Geometry check sheet. Reference: the model listing, model coordinates, mm. Face numbers are marked on the shaded views. A direction names the side the tool comes from. Give positions to 0.01 mm unless a question says otherwise; leave off trailing zeros. Loops run counter-clockwise (first coordinate to the right, second up) from the corner with the lowest first, then second, coordinate; pieces in that order, holes last. Notation, with made-up numbers: (74, 11.5) -> (133, 11.5) arc R22 cw to (133, 20.5) -> close; hole circle Ø3 at (80, 74). An arc over 180 degrees is marked (long way). One line per item, written item: value. Start each with the question number.
(1) Tool access check on the marked faces 1, 2 and 3. Record the directions out of +Z, -Z, +X, -X, +Y, -Y that give a thin tool (end or side, any length) a straight path to the whole face; none if there is none.
(2) Scan lines: line 1 along Z through (x, y) = (25.41, 0.5); line 2 along X through (y, z) = (1.1, 41.59); line 3 along Y through (x, z) = (-19, 34.5). Record each from-to range of solid material in increasing order. Write a range as from..to.
(3) Sectioned sample at C-C, the plane z = -8.5. Record the cut outline in (x, y), then the cut area to 3 significant figures.
(4) Sectioned sample at D-D, the plane x = -7. Record the cut outline in (y, z), then the cut area to 3 significant figures.
(5) Sectioned sample at B-B, the plane x = 25.41. Record the cut outline in (y, z).
(6) Sectioned sample at A-A, the plane z = 41.59. Record the cut outline in (x, y), then the cut area to 3 significant figures.
(7) Gauge pin test, flat ends, axial feed: pin 1 Ø3 at (x, z) = (-9.5, -29) entering from +Y; pin 2 Ø3 at (y, z) = (5, -27.5) entering from +X (3 decimals); pin 3 Ø5 at (x, y) = (-20.5, 6) entering from -Z. Record the tip position at first contact, or that the pin passes through.
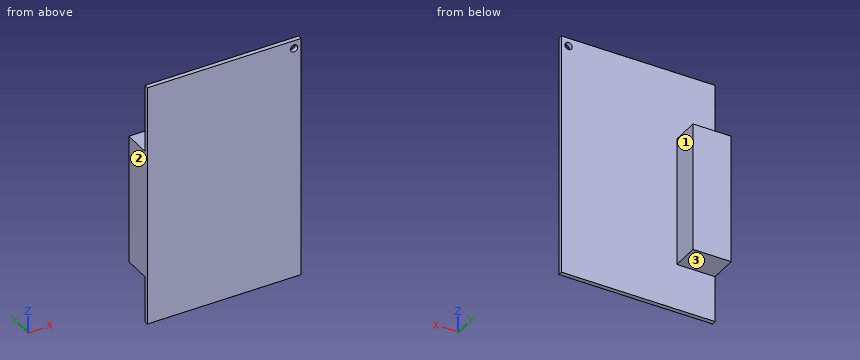
from build123d import *

# Parameters (mm, degrees)
SKETCH_1_W          = 56
SKETCH_1_H          = 89
EXTRUDE_1_DEPTH     = 1.6
SKETCH_2_W          = 13.9249856
SKETCH_2_H          = 47.2640512
EXTRUDE_2_DEPTH     = 10
SKETCH_3_R          = 1.35
CUT_EXTRUDE_1_DEPTH = 10


with BuildPart() as part:
    # 草图1 → 凸台-拉伸1 (new body)
    with BuildSketch(Plane(origin=(0, 0, 0), x_dir=(1, 0, 0), z_dir=(0, 1, 0))):
        Rectangle(SKETCH_1_W, SKETCH_1_H)
    extrude(amount=EXTRUDE_1_DEPTH)

    # 草图2 → 凸台-拉伸2 (add)
    with BuildSketch(Plane(origin=(0, 1.6, 0), x_dir=(1, 0, 0), z_dir=(0, 1, 0))):
        with Locations((-21.0375072, 3.96574336)):
            Rectangle(SKETCH_2_W, SKETCH_2_H)
    extrude(amount=EXTRUDE_2_DEPTH)

    # 草图3 → 切除-拉伸1 (cut)
    with BuildSketch(Plane(origin=(0, 1.6, 0), x_dir=(1, 0, 0), z_dir=(0, 1, 0))):
        with Locations((25.41, -41.59)):
            Circle(SKETCH_3_R)
    extrude(amount=-CUT_EXTRUDE_1_DEPTH, mode=Mode.SUBTRACT)


solid = part.part
Calculated:
1. face 1: +Z, -Z, +X, +Y
1. face 2: +Z, -Z, -X, +Y, -Y
1. face 3: -Z, +X, -X, +Y
2. line 1: z = -44.5..40.24, 42.94..44.5
2. line 2: x = -28..24.06, 26.76..28
2. line 3: y = 0..1.6
3. outline: (-28, 0) -> (28, 0) -> (28, 1.6) -> (-14.08, 1.6) -> (-14.08, 11.6) -> (-28, 11.6) -> close
3. area: 229 mm2
4. outline: (0, -44.5) -> (1.6, -44.5) -> (1.6, 44.5) -> (0, 44.5) -> close
4. area: 142 mm2
5. outline: (0, -44.5) -> (1.6, -44.5) -> (1.6, 40.24) -> (0, 40.24) -> close; (0, 42.94) -> (1.6, 42.94) -> (1.6, 44.5) -> (0, 44.5) -> close
6. outline: (-28, 0) -> (24.06, 0) -> (24.06, 1.6) -> (-28, 1.6) -> close; (26.76, 0) -> (28, 0) -> (28, 1.6) -> (26.76, 1.6) -> close
6. area: 85.3 mm2
7. pin 1: stops at y = 1.6
7. pin 2: stops at x = -14.075
7. pin 3: stops at z = -27.6
